Read the model definition and answer for the solid it produces. Units are mm, in the model's axes. A direction names the side the tool comes from. Coordinates: 2 decimals unless noted, no trailing zeros. Loops run counter-clockwise (first coordinate to the right, second up) from the corner with the lowest first, then second, coordinate; pieces in that order, holes last.
from build123d import *

# Parameters (mm, degrees)
F0_W     = 100
F0_H     = 100
F1_DEPTH = 100
F2_W     = 100
F2_H     = 75.544288
F3_DEPTH = 40
F4_W     = 60
F4_H     = 40
F5_DEPTH = 100.001
F6_DEPTH = 100.001


with BuildPart() as f1:
    # F0 (on Top) → F1 (new body)
    with BuildSketch(Plane.XY):
        Rectangle(F0_W, F0_H)
    extrude(amount=F1_DEPTH)

    # F2 (on face) → F3 (cut)
    with BuildSketch(Plane.XY.offset(100)):
        with Locations((0, -12.227856)):
            Rectangle(F2_W, F2_H)
    extrude(amount=-F3_DEPTH, mode=Mode.SUBTRACT)

    # F4 (on face) → F5 (cut, through all)
    with BuildSketch(Plane.XZ.offset(50)):
        with Locations((-6.015749, 20)):
            Rectangle(F4_W, F4_H)
    extrude(amount=-F5_DEPTH, mode=Mode.SUBTRACT)

    # F4 (on face) → F6 (cut, through all)
    with BuildSketch(Plane.XZ.offset(50)):
        with Locations((-6.015749, 20)):
            Rectangle(F4_W, F4_H)
    extrude(amount=-F6_DEPTH, mode=Mode.SUBTRACT)


solid = f1.part
Q1. Determine the mould class of faces 4 (the face through (37, 1, 0)), 5 (the face through (50, 10, 38)), 6 (the face through (23.984, -1, 20)) for opening direction X: +X half, -X half, draft (parallel to the pull), parting line (faces both ways), or undercut.
Findings below:
face 4: draft
face 5: +X half
face 6: undercut
Q2. A cutting plane is placed at C-C (x = 28). Give the vertices of the cut face in (y, z), then the cut area to 3 significant figures.
Findings below:
outline: (-50, 0) - (50, 0) - (50, 100) - (25.54, 100) - (25.54, 60) - (-50, 60) - close
area: 6,980 mm2
Q3. Which of the six approach directions +Z, -Z, +X, -X, +Y, -Y give full straight-line access (tool end or side, diameter ignored) to faces 1 (the face through (-1, 25.544, 80)), 2 (the face through (-36.016, -1, 20)), 3 (the face through (-50, 10, 38))?
Findings below:
face 1: +Z, +X, -X, -Y
face 2: -Z, +Y, -Y
face 3: +Z, -Z, -X, +Y, -Y
Q4. Straight lines are drawn through the part: probe 1 along X at (y, z) = (-29.5, 18); probe 2 along Z at (x, y) = (-27.5, 18); probe 3 along Y at (x, z) = (2, 69.5). For each, find the intervals that lie inside material, in ascending order.
Findings below:
probe 1: x = -50 to -36.02, 23.98 to 50
probe 2: z = 40 to 60
probe 3: y = 25.54 to 50
Q5. A cutting plane is placed at D-D (z = 63). Give the vertices of the cut face in (x, y), then the cut area to 3 significant figures.
Findings below:
outline: (-50, 25.54) - (50, 25.54) - (50, 50) - (-50, 50) - close
area: 2,450 mm2
Q6. Flat-ended cylindrical pins translate along their axes: pin 1 Ø5 at (x, y) = (-16.5, -15) entering from +Z; pin 2 Ø18 at (x, y) = (8.5, -21.5) entering from -Z. Find the tip coordinate at first contact, or state that the pin passes through.
Findings below:
pin 1: stops at z = 60
pin 2: stops at z = 40
Q7. A cutting plane is placed at A-A (z = 33). Give the vertices of the cut face in (x, y), then the cut area to 3 significant figures.
Findings below:
outline: (-50, -50) - (-36.02, -50) - (-36.02, 50) - (-50, 50) - close; (23.98, -50) - (50, -50) - (50, 50) - (23.98, 50) - close
area: 4,000 mm2
Q8. A cutting plane is placed at B-B (y = 3). Give the vertices of the cut face in (x, z), then the cut area to 3 significant figures.
Findings below:
outline: (-50, 0) - (-36.02, 0) - (-36.02, 40) - (23.98, 40) - (23.98, 0) - (50, 0) - (50, 60) - (-50, 60) - close
area: 3,600 mm2
